Autodesk Inventor part; units mm, degrees
ref_plane "YZ Plane" through (0, 0, 0) normal (1, 0, 0) x (0, 1, 0)
ref_plane "XZ Plane" through (0, 0, 0) normal (0, 1, 0) x (-1, 0, 0)
ref_plane "XY Plane" through (0, 0, 0) normal (0, 0, 1) x (1, 0, 0)
sketch "Sketch1" plane through (0, 0, 0) normal (0, 1, 0) x (-1, 0, 0)
  line L0 (-7.25, 7.25) -> (7.25, 7.25)
  line L1 (7.25, 7.25) -> (7.25, -7.25)
  line L2 (7.25, -7.25) -> (-7.25, -7.25)
  line L3 (-7.25, -7.25) -> (-7.25, 7.25)
  line L4 (-7.25, 7.25) -> (7.25, -7.25) construction
  line L5 (7.25, 7.25) -> (-7.25, -7.25) construction
  point P0 (0, 0)
  dimension "d0" = 14.5
  dimension "d1" = 14.5
extrude "Extrusion1" add sketch "Sketch1" along normal blind 76.2
sketch "Sketch2" plane through (0, 76.2, 0) normal (0, 1, 0) x (1, 0, 0)
  line L0 (10, -10) -> (-10, -10)
  line L1 (-10, -10) -> (-10, 10)
  line L2 (-10, 10) -> (10, 10)
  line L3 (10, 10) -> (10, -10)
  line L4 (10, -10) -> (-10, 10) construction
  line L5 (-10, -10) -> (10, 10) construction
  point P0 (0, 0)
  dimension "d4" = 20
  dimension "d5" = 20
extrude "Extrusion2" add sketch "Sketch2" along normal blind 5
sketch "Sketch3" plane through (0, 81.2, 0) normal (0, 1, 0) x (1, 0, 0)
  line L0 (7.5, -7.5) -> (-7.5, -7.5)
  line L1 (-7.5, -7.5) -> (-7.5, 7.5)
  line L2 (-7.5, 7.5) -> (7.5, 7.5)
  line L3 (7.5, 7.5) -> (7.5, -7.5)
  line L4 (7.5, -7.5) -> (-7.5, 7.5) construction
  line L5 (-7.5, -7.5) -> (7.5, 7.5) construction
  line L6 (10, -10) -> (-10, -10)
  line L7 (-10, -10) -> (-10, 10)
  line L8 (-10, 10) -> (10, 10)
  line L9 (10, 10) -> (10, -10)
  line L10 (10, -10) -> (-10, 10) construction
  line L11 (-10, -10) -> (10, 10) construction
  point P0 (0, 0)
  dimension "d8" = 15
  dimension "d9" = 15
extrude "Extrusion3" add sketch "Sketch3" along normal blind 76.2
sketch "Sketch4" plane through (10, 76.2, 10) normal (1, 0, 0) x (0, 0, -1)
  line L0 (20, 0) -> (20, 81.2)
  line L1 (15, 81.2) -> (15, 0)
  line L2 (0, 0) -> (20, 0)
  line L3 (15, 81.2) -> (13, 81.2)
  line L4 (17.5, 81.2) -> (2.5, 81.2)
  line L5 (13, 81.2) -> (13, 0)
  line L6 (13, 0) -> (15, 0)
  line L7 (20, 81.2) -> (0, 81.2)
  point P0 (10, -76.2)
  dimension "d12" = 2
extrude "Extrusion4" add sketch "Sketch4" along normal blind 10 contours L2 L5 L3 L1
sketch "Sketch5" plane through (10, 76.2, -3) normal (0, 0, 1) x (1, 0, 0)
  line L0 (0, 81.2) -> (10, 81.2)
  line L1 (10, 81.2) -> (8, 81.2)
  line L2 (8, 81.2) -> (8, 0)
  line L3 (8, 0) -> (10, 0)
  line L4 (10, 0) -> (10, 81.2)
  point P0 (-10, -76.2)
  dimension "d15" = 2
extrude "Extrusion5" add sketch "Sketch5" along normal blind 8
sketch "Sketch6" plane through (20, 76.2, 10) normal (1, 0, 0) x (0, 0, -1)
  line L0 (5, 81.2) -> (3, 81.2)
  line L1 (3, 81.2) -> (3, 0)
  line L2 (3, 0) -> (5, 0)
  line L3 (5, 0) -> (5, 81.2)
  point P0 (10, -76.2)
  dimension "d18" = 2
extrude "Extrusion6" add sketch "Sketch6" against normal blind 4
sketch "Sketch7" plane through (0, 157.4, 0) normal (0, 1, 0) x (1, 0, 0)
  line L0 (18, 3) -> (18, -5)
  line L1 (18, 3) -> (18, -5)
  line L2 (18, -1) -> (10, -1)
  line L3 (10, 3) -> (10, -10)
  line L4 (10, -10) -> (10, -1)
  line L5 (10, 10) -> (10, -1)
  line L6 (10, 5) -> (20, 5)
  line L7 (10, 3) -> (18, 3)
  line L8 (10, 3) -> (18, 3)
  point P0 (0, 0)
sketch "Sketch8" plane through (0, 76.2, 0) normal (0, -1, 0) x (1, 0, 0)
  line L0 (16, 7) -> (16, 5)
  line L1 (16, 7) -> (16, 5)
  line L2 (18, 5) -> (18, -3)
  line L3 (18, -3) -> (18, 5)
  line L4 (16, 6) -> (16, 1)
  point P0 (0, 0)
  dimension "d21" = 5
sketch "Sketch9" plane through (7.25, 0, 7.25) normal (1, 0, 0) x (0, 0, -1)
  line L0 (0, 0) -> (14.5, 0)
  line L1 (14.5, 0) -> (14.5, 76.2)
  line L2 (14.5, 76.2) -> (0, 76.2)
  line L3 (0, 76.2) -> (0, 0)
  point P0 (7.25, 0)
extrude "Extrusion7" cut sketch "Sketch9" against normal through all
sketch "Sketch10" plane through (0, 76.2, 0) normal (0, -1, 0) x (1, 0, 0)
  line L0 (10, -5) -> (20, -5)
  line L1 (20, -5) -> (20, 7)
  line L2 (20, 7) -> (10, 7)
  line L3 (10, 7) -> (10, -5)
  point P0 (0, 0)
extrude "Extrusion8" cut sketch "Sketch10" against normal through all
sketch "Sketch11" plane through (10, 76.2, 10) normal (1, 0, 0) x (0, 0, -1)
  line L0 (20, 81.2) -> (50, 81.2)
  line L1 (0, 81.2) -> (-30, 81.2)
  line L2 (-30, 81.2) -> (50, 81.2)
  line L3 (50, 81.2) -> (50, 0.1684)
  line L4 (50, 0.1684) -> (-30, 0.1684)
  line L5 (-30, 0.1684) -> (-30, 81.2)
  point P0 (10, -76.2)
  dimension "d26" = 30
  dimension "d27" = 30
extrude "Extrusion9" add sketch "Sketch11" along normal blind 4
sketch "Sketch12" plane through (14, 76.2, 10) normal (1, 0, 0) x (0, 0, -1)
  line L0 (0, 81.2) -> (0, 76.2)
  line L1 (0, 0) -> (0, 81.2)
  line L2 (0, 66.0511) -> (-25, 66.0511)
  line L3 (-30, 81.2) -> (-30, 0.1684)
  line L4 (0, 25.128) -> (45, 25.128)
  line L5 (50, 0.1684) -> (50, 81.2)
  line L6 (31.5529, 0) -> (31.5529, 5)
  line L7 (-25, 76.2) -> (45, 76.2)
  line L8 (45, 76.2) -> (45, 5)
  line L9 (45, 5) -> (-25, 5)
  line L10 (-25, 5) -> (-25, 76.2)
  line L11 (-30, 81.2) -> (50, 81.2)
  line L12 (50, 81.2) -> (50, 0.1684)
  line L13 (50, 0.1684) -> (-30, 0.1684)
  line L14 (-30, 0.1684) -> (-30, 81.2)
  point P0 (10, -76.2)
  dimension "d30" = 5
  dimension "d31" = 25
  dimension "d32" = 45
  dimension "d33" = 5
extrude "Extrusion10" add sketch "Sketch12" along normal blind 15 contours L11 L5 L13 L6 L9 L8 L7 L0 | L0 L7 L10 L9 L1 L13 L3 L11 | L1 L9 L6 L13
properties part number "CouterWeightLink"
CAD build for the part. Positions are in the model's coordinates, mm. A direction names the side the tool comes from. Round coordinates to 2 decimals unless told otherwise and drop trailing zeros. Write each loop counter-clockwise with the first axis right and the second up, starting at its lowest first coordinate (ties: lowest second). Pieces come first, ordered by that corner, then holes.
(1) Slice it at D-D, the plane x = -4.5. Write the cut outline in (y, z), and give its area (3 significant figures).
(2) Slice it at B-B, the plane y = 103. Write the cut outline in (x, z), and give its area (3 significant figures).
(3) Drop flat-ended pins along their axis: P1, Ø12, axis at x = -0.5, y = 135.5, coming from the -Z side; P2, Ø15, axis at y = 106, z = 30.5, coming from the -X side; P3, Ø12, axis at x = -1, y = 128.5, coming from the +Z side. Give the stop position or say it passes through.
(4) Slice it at A-A, the plane x = 23. Write the cut outline in (y, z), and give its area (3 significant figures).
(5) Probe line 1 along Z through (x, y) = (3, 91); line 2 along Y through (x, z) = (20, -9); line 3 along Z through (x, y) = (26, 116). List the from-to ranges inside material, lowest first.
(6) Slice it at C-C, the plane z = 21.5. Write the cut outline in (x, y).
(7) Mould opens along X. For faces 4 (the face through (10, 117, -25)), 5 (the face through (-7.5, 119, 0)), 6 (the face through (21, 152.4, 0)) say: pulls with the +X half, pulls with the -X half, needs draft (parallel to the pull), parting line crosses it, or undercut.
(8) 3-axis set-ups, long thin cutter, end or side, ignore diameter. For faces 1 (the face through (0, 116, 10)), 2 (the face through (7.5, 119, 0)), 3 (the face through (21, 117, -35)): which of +Z, -Z, +X, -X, +Y, -Y reach the whole face in a straight line?
From the geometry:
1. outline: (76.2, -10) - (157.4, -10) - (157.4, -7.5) - (81.2, -7.5) - (81.2, 7.5) - (157.4, 7.5) - (157.4, 10) - (76.2, 10) - close
1. area: 481 mm2
2. outline: (-10, -10) - (10, -10) - (10, -40) - (29, -40) - (29, -35) - (14, -35) - (14, 35) - (29, 35) - (29, 40) - (10, 40) - (10, 10) - (-10, 10) - close; hole (-7.5, -7.5) - (7.5, -7.5) - (7.5, 7.5) - (-7.5, 7.5) - close
2. area: 645 mm2
3. P1: stops at z = -10
3. P2: stops at x = 10
3. P3: stops at z = 10
4. outline: (76.37, -40) - (157.4, -40) - (157.4, 40) - (76.37, 40) - close; hole (81.2, -35) - (152.4, -35) - (152.4, 35) - (81.2, 35) - close
4. area: 1,500 mm2
5. line 1: z = -10 to -7.5, 7.5 to 10
5. line 2: y = 76.37 to 81.2, 152.4 to 157.4
5. line 3: z = -40 to -35, 35 to 40
6. outline: (10, 76.37) - (29, 76.37) - (29, 81.2) - (14, 81.2) - (14, 152.4) - (29, 152.4) - (29, 157.4) - (10, 157.4) - close
7. face 4: pulls with the -X half
7. face 5: undercut
7. face 6: needs draft
8. face 1: +Z, -X, +Y, -Y
8. face 2: +Y
8. face 3: +X
